Geometry check sheet. Reference: drawing and pictorial views, mm from the part's lowest x, y, z. Coordinates: 2 decimals unless noted, no trailing zeros. Write each loop counter-clockwise with the first axis right and the second up, starting at its lowest first coordinate (ties: lowest second). Pieces come first, ordered by that corner, then holes. Notation, with made-up numbers: (52, 32.25) -> (102, 32.25) arc R10 ccw to (102, 42.25) -> close; hole circle Ø5 at (-31.75, 63). An arc over 180 degrees is marked (long way). Use a Markdown table: item, result.
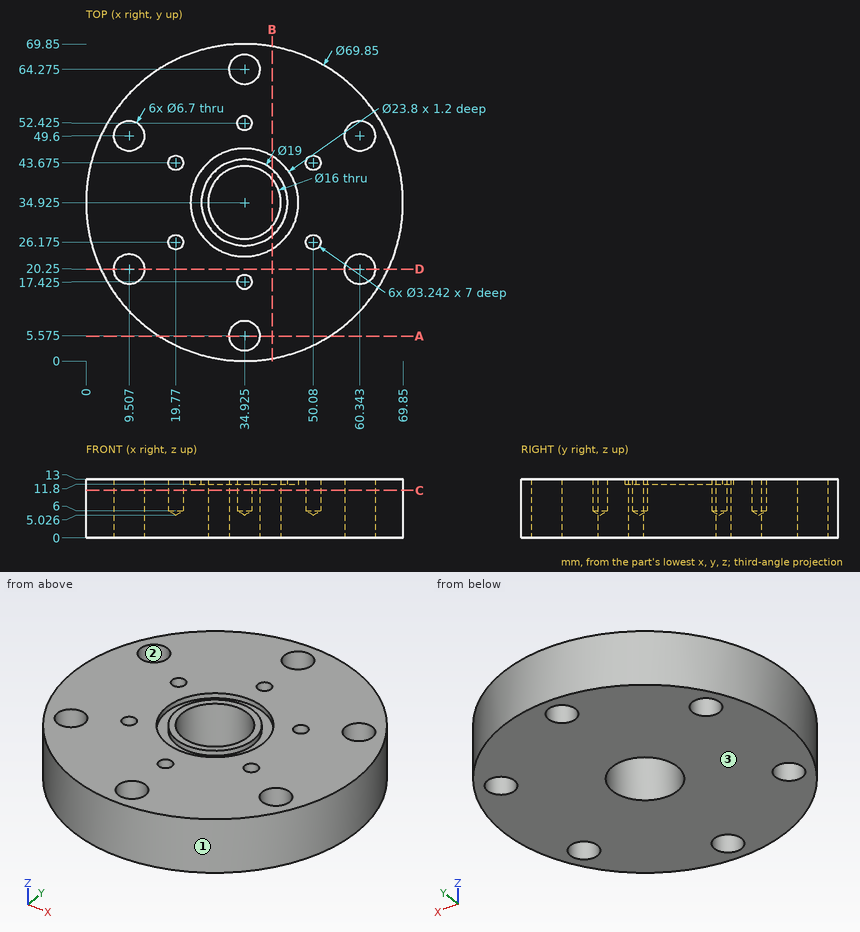
Item 1: Section check A-A on y = 5.5. Record the boundary of the cut face in (x, z).
Answer block:
| item | result |
|---|---|
| outline | (16.11, 0) -> (31.58, 0) -> (31.58, 13) -> (16.11, 13) -> close; (38.27, 0) -> (53.74, 0) -> (53.74, 13) -> (38.27, 13) -> close |
Item 2: Thickness scan on L1, parallel to X at y = 17.5, z = 3 (1 decimal); L2, parallel to X at y = 20.25, z = 6; L3, parallel to Y at x = 60.5, z = 6.75 (1 decimal). Record the ranges inside material, lowest first. Write a range as [from, to].
Answer block:
| item | result |
|---|---|
| L1 | x = [4.7, 7.6], [11.4, 58.4], [62.3, 65.2] |
| L2 | x = [3.23, 6.16], [12.86, 56.99], [63.69, 66.62] |
| L3 | y = [11.1, 16.9], [23.6, 46.3], [52.9, 58.7] |
Item 3: Section check C-C on z = 10.5. Count the separate pieces of the cut face and the enclosed holes in it, then the cut area to 3 significant figures.
Answer block:
| item | result |
|---|---|
| separate pieces | 1 |
| enclosed holes | 13 |
| area | 3,370 mm^2 |
Item 4: Mould release check, pull along X, two halves, no side actions. Record for the marked faces 1, 2 and 3: +X half, -X half, draft (parallel to the pull), parting line (faces both ways), or undercut.
Answer block:
| item | result |
|---|---|
| face 1 | parting line |
| face 2 | undercut |
| face 3 | draft |
Item 5: Section check B-B on x = 41. Record the boundary of the cut face in (y, z).
Answer block:
| item | result |
|---|---|
| outline | (0.53, 0) -> (29.72, 0) -> (29.72, 13) -> (27.62, 13) -> (27.62, 11.8) -> (24.69, 11.8) -> (24.69, 13) -> (0.53, 13) -> close; (40.13, 0) -> (69.32, 0) -> (69.32, 13) -> (45.16, 13) -> (45.16, 11.8) -> (42.23, 11.8) -> (42.23, 13) -> (40.13, 13) -> close |
Item 6: Section check D-D on y = 20.25. Record the boundary of the cut face in (x, z), then the cut area to 3 significant figures.
Answer block:
| item | result |
|---|---|
| outline | (3.23, 0) -> (6.16, 0) -> (6.16, 13) -> (3.23, 13) -> close; (12.86, 0) -> (56.99, 0) -> (56.99, 13) -> (12.86, 13) -> close; (63.69, 0) -> (66.62, 0) -> (66.62, 13) -> (63.69, 13) -> close |
| area | 650 mm^2 |
Item 7: Depth check by flat-ended pin: P1, Ø2, axis at x = 43, z = 10, coming from the -Y side; P2, Ø5, axis at x = 50.08, y = 43.68, coming from the +Z side; P3, Ø4, axis at x = 60.34, y = 20.25, coming from the -Z side; P4, Ø4, axis at y = 62, z = 4, coming from the -X side (1 decimal). Enter the tip coordinate at first touch or a pass-through.
Answer block:
| item | result |
|---|---|
| P1 | stops at y = 0.72 |
| P2 | stops at z = 13 |
| P3 | passes through |
| P4 | stops at x = 10.6 |
